Verification items for the finished model (mm, model axes). A direction names the side the tool comes from. Coordinates: 2 decimals unless noted, no trailing zeros. Loops run counter-clockwise (first coordinate to the right, second up) from the corner with the lowest first, then second, coordinate; pieces in that order, holes last.
Q1. Access from +Z, -Z, +X, -X, +Y, -Y to the whole of each face (thin tool, end or side, straight path). Record for faces 1 (the face through (29.5, -59, 2)), 2 (the face through (73, -104, -2.5)).
Q2. Mould release check, pull along Y, two halves, no side actions. Record for faces 3 (the face through (112, -7, 3)), 4 (the face through (102, 0, 3)), 5 (the face through (102, -116, 3)), 6 (the face through (80, -6, 6)): +Y half, -Y half, draft (parallel to the pull), parting line (faces both ways), or undercut.
Q3. Sectioned sample at C-C (z = 1.5). Enter the section's corners in (x, y), then the cut area to 3 significant figures.
Q4. Sectioned sample at B-B (y = -40). Enter the section's corners in (x, z).
Q5. Sectioned sample at A-A (x = 92). Enter the section's corners in (y, z), then the cut area to 3 significant figures.
Q6. Material ranges on probe 1 along Y at (x, z) = (200, 4.65); probe 2 along Y at (x, z) = (25, 3.45); probe 3 along X at (y, z) = (-7, -0.65), recorded low to high.
Q7. Go/stop test with flat-tipped pins: P1, Ø3, axis at x = 25, y = -7, coming from the +Z side; P2, Ø1, axis at x = 95, y = -102.5, coming from the +Z side. Record where each tip stops, or that it passes through.
```python
from build123d import *

# Parameters (mm, degrees)
F0_W      = 207
F0_H      = 116
F1_DEPTH  = 6
F2_W      = 167
F2_H      = 102
F3_DEPTH  = 6
F4_R      = 1.75
F5_DEPTH  = 25
F6_W      = 10
F6_H      = 60
F7_DEPTH  = 3
F8_W      = 207
F8_H      = 116
F8_R      = 1.75
F8_W_2    = 167
F8_H_2    = 102
F9_DEPTH  = 2.5
F10_W     = 155
F10_H     = 88
F11_DEPTH = 25
F13_R     = 3
F14_R     = 2


with BuildPart() as f1:
    # F0 (on Top) → F1 (new body)
    with BuildSketch(Plane.XY):
        with Locations((103.5, -58)):
            Rectangle(F0_W, F0_H)
    extrude(amount=F1_DEPTH)

    # F2 (on face) → F3 (cut)
    with BuildSketch(Plane.XY):
        with Locations((113, -58)):
            Rectangle(F2_W, F2_H)
    extrude(amount=F3_DEPTH, mode=Mode.SUBTRACT)

    # F4 (on face) → F5 (cut)
    with BuildSketch(Plane(origin=(0, 0, 0), x_dir=(1, 0, 0), z_dir=(0, 0, -1))):
        with Locations((200, 7)):
            Circle(F4_R)
        with Locations((200, 109)):
            Circle(F4_R)
        with Locations((25, 109)):
            Circle(F4_R)
        with Locations((25, 7)):
            Circle(F4_R)
    extrude(amount=-F5_DEPTH, mode=Mode.SUBTRACT)

    # F6 (on face) → F7 (cut)
    with BuildSketch(Plane.XY.offset(6)):
        with Locations((24.5, -58)):
            Rectangle(F6_W, F6_H)
    extrude(amount=-F7_DEPTH, mode=Mode.SUBTRACT)

    # F8 (on face) → F9 (join)
    with BuildSketch(Plane(origin=(0, 0, 0), x_dir=(1, 0, 0), z_dir=(0, 0, -1))):
        with Locations((103.5, 58)):
            Rectangle(F8_W, F8_H)
        with Locations((25, 7)):
            Circle(F8_R, mode=Mode.SUBTRACT)
        with Locations((200, 7)):
            Circle(F8_R, mode=Mode.SUBTRACT)
        with Locations((25, 109)):
            Circle(F8_R, mode=Mode.SUBTRACT)
        with Locations((113, 58)):
            Rectangle(F8_W_2, F8_H_2, mode=Mode.SUBTRACT)
        with Locations((200, 109)):
            Circle(F8_R, mode=Mode.SUBTRACT)
        with Locations((113, 58)):
            Rectangle(F8_W_2, F8_H_2)
    extrude(amount=F9_DEPTH)

    # F10 (on face) → F11 (cut)
    with BuildSketch(Plane(origin=(0, 0, -2.5), x_dir=(1, 0, 0), z_dir=(0, 0, -1))):
        with Locations((114.5, 55)):
            Rectangle(F10_W, F10_H)
    extrude(amount=-F11_DEPTH, mode=Mode.SUBTRACT)

    # F13
    f13_edges = [f1.edges().sort_by_distance(p)[0] for p in [
        (207, 0, 1.75),
        (0, 0, 1.75),
        (207, -116, 1.75),
        (0, -116, 1.75),
    ]]
    fillet(f13_edges, radius=F13_R)

    # F14
    f14_edges = [f1.edges().sort_by_distance(p)[0] for p in [
        (0, -58, -2.5),
        (114.5, -99, -2.5),
        (37, -55, -2.5),
        (192, -55, -2.5),
        (114.5, -11, -2.5),
        (103.5, 0, -2.5),
        (206.12132, -0.87868, -2.5),
        (0.87868, -0.87868, -2.5),
        (207, -58, -2.5),
        (0.87868, -115.12132, -2.5),
        (206.12132, -115.12132, -2.5),
        (103.5, -116, -2.5),
    ]]
    fillet(f14_edges, radius=F14_R)


solid = f1.part
```
Geometry check:
1. face 1: +Z
1. face 2: -Z, +X, -X, +Y, -Y
2. face 3: undercut
2. face 4: +Y half
2. face 5: -Y half
2. face 6: draft
3. outline: (0, -113) arc R3 ccw to (3, -116) - (204, -116) arc R3 ccw to (207, -113) - (207, -3) arc R3 ccw to (204, 0) - (3, 0) arc R3 ccw to (0, -3) - close; hole circle Ø3.5 at (25, -109); hole circle Ø3.5 at (25, -7); hole (29.5, -109) - (196.5, -109) - (196.5, -7) - (29.5, -7) - close; hole circle Ø3.5 at (200, -109); hole circle Ø3.5 at (200, -7)
3. area: 6,930 mm2
4. outline: (0, -0.5) arc R2 ccw to (2, -2.5) - (35, -2.5) arc R2 ccw to (37, -0.5) - (37, 0) - (29.5, 0) - (29.5, 3) - (19.5, 3) - (19.5, 6) - (0, 6) - close; (192, -0.5) arc R2 ccw to (194, -2.5) - (205, -2.5) arc R2 ccw to (207, -0.5) - (207, 6) - (196.5, 6) - (196.5, 0) - (192, 0) - close
5. outline: (-116, -0.5) arc R2 ccw to (-114, -2.5) - (-101, -2.5) arc R2 ccw to (-99, -0.5) - (-99, 0) - (-109, 0) - (-109, 6) - (-116, 6) - close; (-11, -0.5) arc R2 ccw to (-9, -2.5) - (-2, -2.5) arc R2 ccw to (0, -0.5) - (0, 6) - (-7, 6) - (-7, 0) - (-11, 0) - close
5. area: 151 mm2
6. probe 1: y = -116 to -110.75, -107.25 to -8.75, -5.25 to 0
6. probe 2: y = -116 to -110.75, -107.25 to -88, -28 to -8.75, -5.25 to 0
6. probe 3: x = 0.01 to 23.25, 26.75 to 198.25, 201.75 to 206.99
7. P1: passes through
7. P2: stops at z = 0
